Autodesk Inventor part; units mm, degrees
ref_plane "YZ Plane" through (0, 0, 0) normal (1, 0, 0) x (0, 1, 0)
ref_plane "XZ Plane" through (0, 0, 0) normal (0, 1, 0) x (-1, 0, 0)
ref_plane "XY Plane" through (0, 0, 0) normal (0, 0, 1) x (1, 0, 0)
sketch "Sketch1" plane through (0, 0, 0) normal (0, 1, 0) x (-1, 0, 0)
  line L0 (-138.1445, 75.4197) -> (-138.1445, 125.4197)
  line L1 (-138.1445, -54.5803) -> (-138.1445, -4.5803)
  line L2 (-118.1445, -74.5803) -> (-68.1445, -74.5803)
  line L3 (1.8555, -74.5803) -> (51.8555, -74.5803)
  line L4 (71.8555, -54.5803) -> (71.8555, -4.5803)
  line L5 (71.8555, 125.4197) -> (71.8555, 75.4197)
  line L6 (51.8555, 145.4197) -> (1.8555, 145.4197)
  line L7 (-68.1445, 145.4197) -> (-118.1445, 145.4197)
  line L8 (51.8555, -74.5803) -> (71.8555, -74.5803)
  line L9 (71.8555, -74.5803) -> (71.8555, -54.5803)
  line L10 (71.8555, -74.5803) -> (-138.1445, -74.5803)
  line L11 (-138.1445, -74.5803) -> (-138.1445, 145.4197)
  line L12 (-138.1445, 145.4197) -> (71.8555, 145.4197)
  line L13 (71.8555, 145.4197) -> (71.8555, -74.5803)
  line L14 (96.8555, -89.5803) -> (96.8555, -99.5803)
  line L15 (96.8555, -99.5803) -> (-163.1445, -99.5803)
  line L16 (-163.1445, -99.5803) -> (-163.1445, 170.4197)
  line L17 (-163.1445, 170.4197) -> (96.8555, 170.4197)
  line L18 (96.8555, 170.4197) -> (96.8555, -99.5803)
  circle A0 centre (-33.1445, 35.4197) radius 7.5
  circle A1 centre (-33.1445, 35.4197) radius 15
  point P0 (0, 0)
  dimension "d37" = 260
  dimension "d38" = 270
  dimension "d39" = 260
  dimension "d40" = 15
  dimension "d41" = 30
extrude "Extrusion2" add sketch "Sketch1" against normal blind 5 contours L0 L11 L12 L7 L6 L13 L5 L4 L9 L8 L3 L10 L2 L1 | A0 | A1
extrude "Extrusion3" add sketch "Sketch1" along normal blind 5 contours L0 L11 L12 L7 L6 L13 L5 L4 L9 L8 L3 L10 L2 L1 | L14 L15 L16 L17 L18 | A0 | A1
extrude "Extrusion4" add sketch "Sketch1" along normal blind 15 contours A0
ref_plane "Work Plane3" through (33.1445, 15, 35.4197) normal (0, 1, 0) x (1, 0, 0)
sketch "Sketch2" plane through (33.1445, 15, 35.4197) normal (0, 1, 0) x (1, 0, 0)
  circle A0 centre (0, 0) radius 15
  point P0 (-33.1445, 35.4197)
  dimension "d53" = 30
extrude "Extrusion6" add sketch "Sketch2" along normal blind 10
properties part number "Part Buttom"
Verification items for the finished model (mm, model axes). Give positions to 0.01 mm unless a question says otherwise; leave off trailing zeros. Write each loop counter-clockwise with the first axis right and the second up, starting at its lowest first coordinate (ties: lowest second). Pieces come first, ordered by that corner, then holes. Notation, with made-up numbers: (12, -29) - (47, -29) arc R28 cw to (47, -8) - close; hole circle Ø7 at (-21, 11.5). An arc over 180 degrees is marked (long way). Put each result on its own line as item: value.
Q1. Section check B-B on x = -23. Record the cut outline in (y, z).
Result:
outline: (-5, -74.58) - (0, -74.58) - (0, -99.58) - (5, -99.58) - (5, 170.42) - (0, 170.42) - (0, 145.42) - (-5, 145.42) - close
Q2. Depth check by flat-ended pin: P1, Ø2.5, axis at y = -3, z = 66.5, coming from the +X side; P2, Ø1, axis at x = -52.5, z = 131.5, coming from the +Y side; P3, Ø4, axis at x = 60, y = -3.5, coming from the +Z side. Enter the tip coordinate at first touch or a pass-through.
Result:
P1: x = 138.14
P2: y = 5
P3: z = 145.42
Q3. Section check C-C on y = 9.5. Record the cut outline in (x, z).
Result:
outline: circle Ø15 at (33.14, 35.42)
Q4. Section check A-A on z = -20. Record the cut outline in (x, y).
Result:
outline: (-96.86, 0) - (-71.86, 0) - (-71.86, -5) - (138.14, -5) - (138.14, 0) - (163.14, 0) - (163.14, 5) - (-96.86, 5) - close
Q5. Mould release check, pull along Y, two halves, no side actions. Record for faces 1 (the face through (35, -5, 37)), 2 (the face through (33, 25, 35)), 3 (the face through (26, 15, 39)), 4 (the face through (18.16, 19.93, 36.08)): released by +Y, released by -Y, zero draft, split by the parting line, or undercut.
Result:
face 1: released by -Y
face 2: released by +Y
face 3: undercut
face 4: zero draft
Q6. Scan lines: probe 1 along Z at (x, y) = (-62, -1); probe 2 along Y at (x, z) = (136.5, 4); probe 3 along X at (y, z) = (-2.25, 139.5). Record each from-to range of solid material in increasing order. Write a range as from..to.
Result:
probe 1: -74.58..145.42
probe 2: -5..5
probe 3: -71.86..138.14
